Design review of the part built by this model. Coordinates are the model's own, in mm. A direction names the side the tool comes from. Coordinates: 2 decimals unless noted, no trailing zeros. Loops run counter-clockwise (first coordinate to the right, second up) from the corner with the lowest first, then second, coordinate; pieces in that order, holes last. Notation, with made-up numbers: (-33, 61.25) -> (2, 61.25) arc R13 ccw to (2, 67.25) -> close; hole circle Ø5 at (-16.5, -5.5). An arc over 180 degrees is marked (long way). Answer in a Markdown table with one row per item.
```python
from build123d import *

# Parameters (mm, degrees)
F0_W     = 12.7
F0_H     = 63.5
F1_DEPTH = 25.4
F2_R     = 4.445
F3_DEPTH = 88.901


with BuildPart() as f1:
    # F0 (on Front) → F1 (new body)
    with BuildSketch(Plane.XZ):
        Polygon((37.03399, -6.35), (44.45, -6.35), (44.45, 6.35), (-44.45, 6.35), (-44.45, -6.35), (-37.03399, -6.35), (-24.33399, -6.35), (24.33399, -6.35), align=None)
        with Locations((30.68399, -38.1)):
            Rectangle(F0_W, F0_H)
        with Locations((-30.68399, -38.1)):
            Rectangle(F0_W, F0_H)
    extrude(amount=F1_DEPTH)

    # F2 (on face) → F3 (cut, through all)
    with BuildSketch(Plane(origin=(-44.45, 0, 0), x_dir=(0, -1, 0), z_dir=(-1, 0, 0))):
        with Locations((12.7, 0)):
            Circle(F2_R)
    extrude(amount=-F3_DEPTH, mode=Mode.SUBTRACT)


solid = f1.part
```
(1) Take a section at D-D on y = -3. Give the boundary of the cut face in (x, z), and give its area (3 significant figures).
Evaluation:
| item | result |
|---|---|
| outline | (-44.45, -6.35) -> (-37.03, -6.35) -> (-37.03, -69.85) -> (-24.33, -69.85) -> (-24.33, -6.35) -> (24.33, -6.35) -> (24.33, -69.85) -> (37.03, -69.85) -> (37.03, -6.35) -> (44.45, -6.35) -> (44.45, 6.35) -> (-44.45, 6.35) -> close |
| area | 2,740 mm² |
(2) Take a section at A-A on y = -12.7. Give the boundary of the cut face in (x, z) (3 decimals).
Evaluation:
| item | result |
|---|---|
| outline | (-44.45, -6.35) -> (-37.034, -6.35) -> (-37.034, -69.85) -> (-24.334, -69.85) -> (-24.334, -6.35) -> (24.334, -6.35) -> (24.334, -69.85) -> (37.034, -69.85) -> (37.034, -6.35) -> (44.45, -6.35) -> (44.45, -4.445) -> (-44.45, -4.445) -> close; (-44.45, 4.445) -> (44.45, 4.445) -> (44.45, 6.35) -> (-44.45, 6.35) -> close |
(3) Take a section at B-B on z = 0. Give the boundary of the cut face in (x, y) (3 decimals).
Evaluation:
| item | result |
|---|---|
| outline | (-44.45, -25.4) -> (44.45, -25.4) -> (44.45, -17.145) -> (-44.45, -17.145) -> close; (-44.45, -8.255) -> (44.45, -8.255) -> (44.45, 0) -> (-44.45, 0) -> close |
(4) For pin 1 (6 mm diameter, centred on x = 42, y = -16, fed in from -Z); pin 2 (12.5 mm diameter, centred on y = -13, z = -43.5, fed in from +X); pin 3 (4 mm diameter, centred on y = -15, z = -52.5, fed in from -X), all flat-tipped, find the tip position at first contact; note any pin that passes through.
Evaluation:
| item | result |
|---|---|
| pin 1 | stops at z = -6.35 |
| pin 2 | stops at x = 37.03 |
| pin 3 | stops at x = -37.03 |
(5) To check wall thickness, follow probe 1 along Z at (x, y) = (17.5, -12.7) (3 decimals); probe 2 along X at (y, z) = (-11.25, -11.5); probe 3 along Z at (x, y) = (20, -5.25). State the ranges of each line that lie inside material, in increasing order.
Evaluation:
| item | result |
|---|---|
| probe 1 | z = -6.35 to -4.445, 4.445 to 6.35 |
| probe 2 | x = -37.03 to -24.33, 24.33 to 37.03 |
| probe 3 | z = -6.35 to 6.35 |
(6) Draft analysis for pull direction X (two halves, no side actions). For faces 5 (the flat face through (41, -13, -6.35)), 6 (the flat face through (0, -13, -6.35)), 7 (the flat face through (-44.45, -10, -4)), state which applies: pulls with the +X half, pulls with the -X half, needs draft (parallel to the pull), parting line crosses it, or undercut.
Evaluation:
| item | result |
|---|---|
| face 5 | needs draft |
| face 6 | undercut |
| face 7 | pulls with the -X half |
(7) Tool access review of faces 1 (the flat face through (24.334, -13, -39)), 2 (the flat face through (44.45, -10, 4)), 3 (the flat face through (37.034, -13, -39)), 4 (the flat face through (-41, -13, -6.35)): name each direction out of +Z, -Z, +X, -X, +Y, -Y from which nothing blocks a thin tool from reaching the whole face with its end or side.
Evaluation:
| item | result |
|---|---|
| face 1 | -Z, +Y, -Y |
| face 2 | +Z, -Z, +X, +Y, -Y |
| face 3 | -Z, +X, +Y, -Y |
| face 4 | -Z, -X, +Y, -Y |
(8) Take a section at C-C on x = 25.5. Give the boundary of the cut face in (y, z) (3 decimals).
Evaluation:
| item | result |
|---|---|
| outline | (-25.4, -69.85) -> (0, -69.85) -> (0, 6.35) -> (-25.4, 6.35) -> close; hole circle Ø8.89 at (-12.7, 0) |
